Geometry: see drawing. Coordinates: mm, zero at the bounding-box minimum. Round coordinates to 2 decimals unless told otherwise and drop trailing zeros. Loops run counter-clockwise (first coordinate to the right, second up) from the corner with the lowest first, then second, coordinate; pieces in that order, holes last. Notation, with made-up numbers: (-40, 54.25) - (-26, 54.25) arc R17 cw to (-26, 81.25) - close; hole circle Ø10 at (68.5, 3.25). An arc over 180 degrees is marked (long way). Return JSON: item names as keys, results as strings. Group by question number.
1. Section B-B on y = 1. Return loops of the section in (x, z), and give its area (3 significant figures).
2. Section A-A on x = 6. Return loops of the section in (y, z).
3. Material intervals for probe 1 along Z at (x, y) = (4.5, 3.75); probe 2 along Z at (x, y) = (3.75, 6); probe 3 along Y at (x, z) = (21.5, 49.5), sorted ascending.
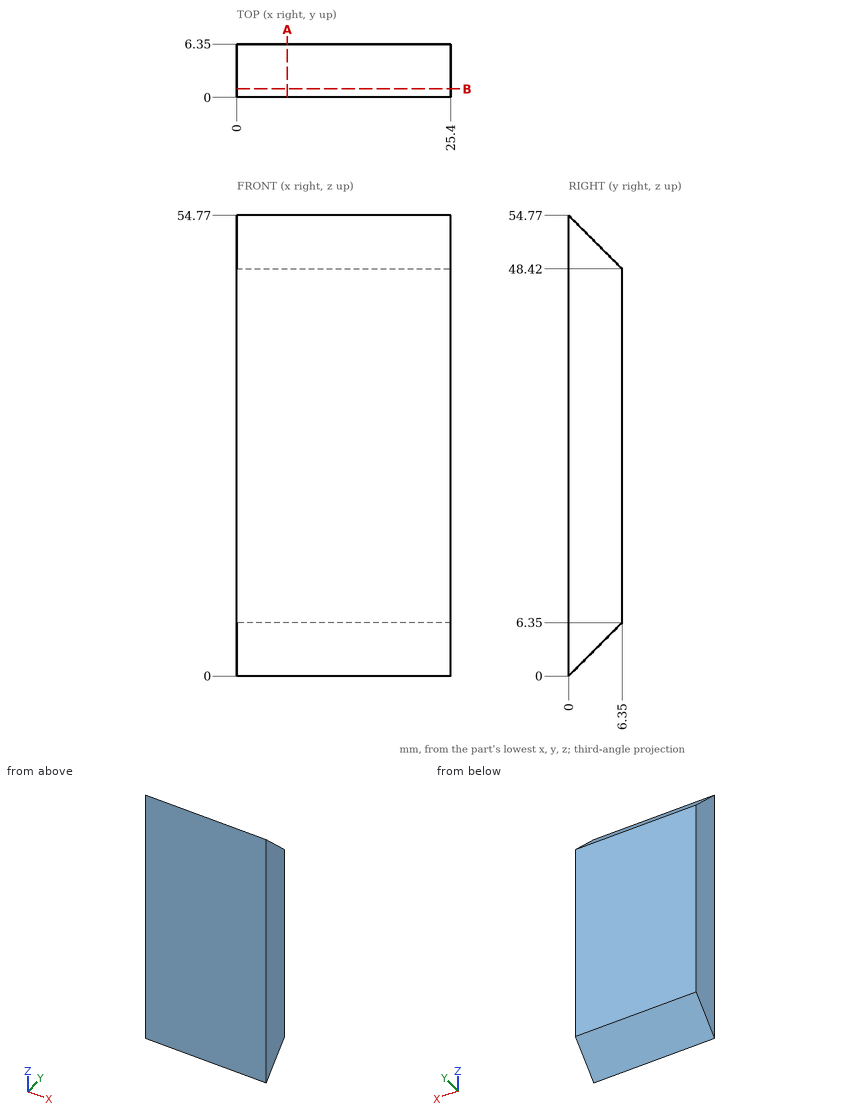
Taken from the geometry:
{
 "1": {"outline": "(0, 1) - (25.4, 1) - (25.4, 53.77) - (0, 53.77) - close", "area": "1,340 mm2"},
 "2": {"outline": "(0, 0) - (6.35, 6.35) - (6.35, 48.42) - (0, 54.77) - close"},
 "3": {"probe 1": "3.75 to 51.02", "probe 2": "6 to 48.77", "probe 3": "0 to 5.27"}
}
